from build123d import *

# Parameters (mm, degrees)
F0_R     = 18.034
F0_R_2   = 14.859
F1_DEPTH = 12.7
F2_R     = 2.54
F3_DEPTH = 50.8
F4_DEPTH = 50.8


with BuildPart() as f1:
    # F0 (on Top) → F1 (new body)
    with BuildSketch(Plane.XY):
        Circle(F0_R)
        Circle(F0_R_2, mode=Mode.SUBTRACT)
    extrude(amount=F1_DEPTH)

    # F2 (on Front) → F3 (cut)
    with BuildSketch(Plane.XZ):
        with Locations((0, 6.187824)):
            Circle(F2_R)
    extrude(amount=-F3_DEPTH, mode=Mode.SUBTRACT)

    # F2 (on Front) → F4 (cut)
    with BuildSketch(Plane.XZ):
        with Locations((0, 6.187824)):
            Circle(F2_R)
    extrude(amount=F4_DEPTH, mode=Mode.SUBTRACT)


solid = f1.part
Source: CAD feature listing. Evaluate the final solid. Frame: model axes, mm. Give positions to 0.01 mm unless a question says otherwise; leave off trailing zeros. Loops run counter-clockwise (first coordinate to the right, second up) from the corner with the lowest first, then second, coordinate; pieces in that order, holes last. Notation, with made-up numbers: (-27.5, 41) -> (-3.5, 41) arc R23 ccw to (-3.5, 61) -> close; hole circle Ø7 at (66, 32). An arc over 180 degrees is marked (long way). Use a Markdown table: item, result. Add a question column.
1) Section query C-C, the plane z = 6.75. Return the cut outline in (x, y), then the cut area to 3 significant figures.
2) Section query B-B, the plane x = 0. Return the cut outline in (y, z).
3) First-contact query: pin 1 (2 mm diameter, centred on x = 2, z = 9.5, fed in from +Y); pin 2 (6 mm diameter, centred on x = 0, z = 6.19, fed in from -Y); pin 3 (3 mm diameter, centred on y = -2, z = 4.5, fed in from -X); pin 4 (1.5 mm diameter, centred on y = 11, z = 8.5, fed in from -X). Flat tips, straight axial feed; report the tip coordinate or a pass-through.
4) Section query A-A, the plane y = 0. Return the cut outline in (x, z).
5) Pull-direction query (X, two-part tool) for faces 1 (the face through (3, 15, 12.7)), 2 (the face through (-0.331, 16.313, 8.706)), 3 (the face through (-3.909, -17.605, 6.261)); classes: +X half, -X half, draft (parallel to the pull), parting line (faces both ways), or undercut.
6) Section query D-D, the plane z = 9.75. Return the cut outline in (x, y).
7) Line query: line 1 along Z through (x, y) = (0, -15.9); line 2 along X through (y, z) = (-12, 1.5); line 3 along X through (y, z) = (11.5, 6). Output: solid intervals per line, ascending. Write a range as [from, to].
Numbers:
| question | item | result |
|---|---|---|
| 1 | outline | (-2.48, -17.86) -> (-2.48, -14.65) arc R14.86 cw to (-2.48, 14.65) -> (-2.48, 17.86) arc R18.03 ccw to start; (2.48, -17.86) arc R18.03 ccw to (2.48, 17.86) -> (2.48, 14.65) arc R14.86 cw to (2.48, -14.65) -> close |
| 1 | area | 297 mm2 |
| 2 | outline | (-18.03, 0) -> (-14.86, 0) -> (-14.86, 3.65) -> (-18.03, 3.65) -> close; (-18.03, 8.73) -> (-14.86, 8.73) -> (-14.86, 12.7) -> (-18.03, 12.7) -> close; (14.86, 0) -> (18.03, 0) -> (18.03, 3.65) -> (14.86, 3.65) -> close; (14.86, 8.73) -> (18.03, 8.73) -> (18.03, 12.7) -> (14.86, 12.7) -> close |
| 3 | pin 1 | stops at y = 18.01 |
| 3 | pin 2 | stops at y = -18.03 |
| 3 | pin 3 | stops at x = -18.03 |
| 3 | pin 4 | stops at x = -14.84 |
| 4 | outline | (-18.03, 0) -> (-14.86, 0) -> (-14.86, 12.7) -> (-18.03, 12.7) -> close; (14.86, 0) -> (18.03, 0) -> (18.03, 12.7) -> (14.86, 12.7) -> close |
| 5 | face 1 | draft |
| 5 | face 2 | undercut |
| 5 | face 3 | parting line |
| 6 | outline | circle Ø36.07 at (0, 0); hole circle Ø29.72 at (0, 0) |
| 7 | line 1 | z = [0, 3.65], [8.73, 12.7] |
| 7 | line 2 | x = [-13.46, -8.76], [8.76, 13.46] |
| 7 | line 3 | x = [-13.89, -9.41], [9.41, 13.89] |
